Verification items for the finished model (mm, model axes). A direction names the side the tool comes from. Round coordinates to 2 decimals unless told otherwise and drop trailing zeros. Loops run counter-clockwise (first coordinate to the right, second up) from the corner with the lowest first, then second, coordinate; pieces in that order, holes last.
from build123d import *

# Parameters (mm, degrees)
CROQUIS1_R                     = 21.825
SALIENTE_EXTRUIR1_DEPTH        = 4.5
CROQUIS2_R                     = 2.75
SALIENTE_EXTRUIR2_DEPTH        = 12
TALADRO_DE_MARGEN_PARA_M121_D  = 13.5
SALIENTE_EXTRUIR3_DEPTH        = 12
CROQUIS8_R                     = 1.7
CORTAR_EXTRUIR1_DEPTH          = 16.5
MATRIZC1_COUNT                 = 3
TALADRO_DE_MARGEN_PARA_M2_51_D = 2.9
SALIENTE_EXTRUIR5_DEPTH        = 4.5
MATRIZC2_COUNT                 = 3
CROQUIS12_R                    = 2.875
CORTAR_EXTRUIR2_DEPTH          = 2.2
CROQUIS13_R                    = 3.1
CORTAR_EXTRUIR3_DEPTH          = 2


with BuildPart() as part:
    # Croquis1 → Saliente-Extruir1 (new body)
    with BuildSketch(Plane(origin=(0, 0, 0), x_dir=(1, 0, 0), z_dir=(0, 1, 0))):
        Circle(CROQUIS1_R)
    extrude(amount=SALIENTE_EXTRUIR1_DEPTH)

    # Croquis2 → Saliente-Extruir2 (add)
    with BuildSketch(Plane(origin=(0, 4.5, 0), x_dir=(1, 0, 0), z_dir=(0, 1, 0))):
        with Locations((0, 15)):
            Circle(CROQUIS2_R)
        with Locations((12.990381057, -7.5)):
            Circle(CROQUIS2_R)
        with Locations((-12.990381057, -7.5)):
            Circle(CROQUIS2_R)
    extrude(amount=SALIENTE_EXTRUIR2_DEPTH)

    # Taladro de margen para M121 (through all)
    with Locations(Plane(origin=(0, 4.5, 0), x_dir=(1, 0, 0), z_dir=(0, 1, 0))):
        with Locations((0, 0)):
            Hole(TALADRO_DE_MARGEN_PARA_M121_D / 2)

    # Croquis5 → Saliente-Extruir3 (add)
    with BuildSketch(Plane(origin=(0, 4.5, 0), x_dir=(1, 0, 0), z_dir=(0, 1, 0))):
        with BuildLine():
            ThreePointArc((-7.642674188, 4.4125), (-11.035446071, 10.994501306), (-11.800237164, 18.359875487))
            ThreePointArc((-11.800237164, 18.359875487), (-18.901004438, 10.9125), (-21.800237164, 1.039367411))
            ThreePointArc((-21.800237164, 1.039367411), (-15.039240468, 4.059725986), (-7.642674188, 4.4125))
        make_face()
    saliente_extruir3 = extrude(amount=SALIENTE_EXTRUIR3_DEPTH)

    # Croquis8 → Cortar-Extruir1 (cut)
    with BuildSketch(Plane(origin=(0, 16.5, 0), x_dir=(1, 0, 0), z_dir=(0, 1, 0))):
        with Locations((-14.722431864, 8.5)):
            Circle(CROQUIS8_R)
    cortar_extruir1 = extrude(amount=-CORTAR_EXTRUIR1_DEPTH, mode=Mode.SUBTRACT)

    # MatrizC1: Saliente-Extruir3, Cortar-Extruir1 ×3 about axis
    matrizc1_axis = Axis((0, 0, 0), (0, 1, 0))
    for i in range(1, MATRIZC1_COUNT):
        add(saliente_extruir3.rotate(matrizc1_axis, i * 360 / MATRIZC1_COUNT))
        add(cortar_extruir1.rotate(matrizc1_axis, i * 360 / MATRIZC1_COUNT), mode=Mode.SUBTRACT)

    # Taladro de margen para M2.51 (through all)
    with Locations(Plane(origin=(0, 16.5, 0), x_dir=(1, 0, 0), z_dir=(0, 1, 0))):
        with Locations((12.990381057, -7.5), (-12.990381057, -7.5), (0, 15)):
            Hole(TALADRO_DE_MARGEN_PARA_M2_51_D / 2)

    # Croquis11 → Saliente-Extruir5 (add)
    with BuildSketch(Plane.XZ):
        with BuildLine():
            ThreePointArc((-10, 19.399242898), (-18.901004438, 10.9125), (-21.800237164, -1.039367411))
            ThreePointArc((-21.800237164, -1.039367411), (-23.615858472, 13.634622246), (-10, 19.399242898))
        make_face()
    saliente_extruir5 = extrude(amount=-SALIENTE_EXTRUIR5_DEPTH)

    # MatrizC2: Saliente-Extruir5 ×3 about axis
    matrizc2_axis = Axis((0, 0, 0), (0, 1, 0))
    for i in range(1, MATRIZC2_COUNT):
        add(saliente_extruir5.rotate(matrizc2_axis, i * 360 / MATRIZC2_COUNT))

    # Croquis12 → Cortar-Extruir2 (cut)
    with BuildSketch(Plane.XZ):
        with Locations((-12.990381057, 7.5)):
            Circle(CROQUIS12_R)
        with Locations((12.990381057, 7.5)):
            Circle(CROQUIS12_R)
        with Locations((0, -15)):
            Circle(CROQUIS12_R)
    extrude(amount=-CORTAR_EXTRUIR2_DEPTH, mode=Mode.SUBTRACT)

    # Croquis13 → Cortar-Extruir3 (cut)
    with BuildSketch(Plane(origin=(0, 16.5, 0), x_dir=(1, 0, 0), z_dir=(0, 1, 0))):
        with Locations((0, -17)):
            Circle(CROQUIS13_R)
        with Locations((-14.722431864, 8.5)):
            Circle(CROQUIS13_R)
        with Locations((14.722431864, 8.5)):
            Circle(CROQUIS13_R)
    extrude(amount=-CORTAR_EXTRUIR3_DEPTH, mode=Mode.SUBTRACT)


solid = part.part
1. Section check C-C (z = -6). Enter the section's corners in (x, y).
2. Tool access check on faces 1 (the face through (-13.614, 1.085, 4.693)), 2 (the face through (-15.141, 10.416, -4.035)), 3 (the face through (-0.221, 7.352, 15.314)). Record the directions out of +Z, -Z, +X, -X, +Y, -Y that give a thin tool (end or side, any length) a straight path to the whole face; none if there is none.
3. Release check for a two-part mould opening along X. For faces 4 (the face through (-17.4, 16.5, -10.4)), 5 (the face through (1.46, 2.22, 6.59)), 6 (the face through (-13.15, 7.35, -7.85)) record: released by +X, released by -X, zero draft, split by the parting line, or undercut.
4. Section check A-A (z = 7.5). Enter the section's corners in (x, y).
5. Gauge pin test, flat ends, axial feed: P1, Ø5, axis at x = -13.5, z = -10, coming from the +Y side; P2, Ø8, axis at x = 8.5, y = 4.5, coming from the -Z side; P3, Ø5, axis at x = -14.72, z = -8.5, coming from the +Y side; P4, Ø1.5, axis at x = 6, z = -3.5, coming from the +Y side. Record the tip position at first contact, or that the pin passes through.
6. Section check D-D (x = 21). Enter the section's corners in (y, z).
7. Section check B-B (y = 6.75). Give the number of separate pieces and of enclosed holes in the cut face, then the cut area to 3 significant figures.
8. Scan lines: L1, parallel to Z at x = 1.5, y = 5.75; L2, parallel to Y at x = 11, z = 15; L3, parallel to X at y = 6.75, z = -11. Record each from-to range of solid material in increasing order.
Taken from the geometry:
1. outline: (-20.98, 0) - (-3.09, 0) - (-3.09, 4.5) - (-8.76, 4.5) - (-8.76, 16.5) - (-12.89, 16.5) - (-12.89, 14.5) - (-16.56, 14.5) - (-16.56, 16.5) - (-20.98, 16.5) - close; (3.09, 0) - (20.98, 0) - (20.98, 16.5) - (16.56, 16.5) - (16.56, 14.5) - (12.89, 14.5) - (12.89, 16.5) - (8.76, 16.5) - (8.76, 4.5) - (3.09, 4.5) - close
2. face 1: -Y
2. face 2: +Y
2. face 3: +Y, -Y
3. face 4: zero draft
3. face 5: undercut
3. face 6: undercut
4. outline: (-25.26, 0) - (-15.87, 0) - (-15.87, 2.2) - (-14.44, 2.2) - (-14.44, 16.5) - (-15.74, 16.5) - (-15.74, 4.5) - (-25.26, 4.5) - close; (-11.54, 2.2) - (-10.12, 2.2) - (-10.12, 0) - (10.12, 0) - (10.12, 2.2) - (11.54, 2.2) - (11.54, 16.5) - (10.24, 16.5) - (10.24, 4.5) - (-10.24, 4.5) - (-10.24, 16.5) - (-11.54, 16.5) - close; (14.44, 2.2) - (15.87, 2.2) - (15.87, 0) - (25.26, 0) - (25.26, 4.5) - (15.74, 4.5) - (15.74, 16.5) - (14.44, 16.5) - close
5. P1: stops at y = 16.5
5. P2: stops at z = -26.41
5. P3: stops at y = 14.5
5. P4: stops at y = 4.5
6. outline: (0, -5.94) - (16.5, -5.94) - (16.5, -1.57) - (4.5, -1.57) - (4.5, 16.79) - (0, 16.79) - close
7. separate pieces: 6
7. enclosed holes: 6
7. area: 359 mm2
8. L1: z = -17.3 to -12.7, 11.79 to 16.2, 17.8 to 21.77
8. L2: y = 0 to 4.5
8. L3: x = -18.85 to -11.04, 11.04 to 18.85
